Check sheet for the drawn part. Datum: minimum x, y, z corner. Units: mm. A direction names the side the tool comes from. Coordinates: 2 decimals unless noted, no trailing zeros. Write each loop counter-clockwise with the first axis right and the second up, starting at its lowest first coordinate (ties: lowest second). Pieces come first, ordered by that corner, then holes. Notation, with made-up numbers: M 84,11.5 L 107,11.5 A11 cw 107,15.5 Z; hole C 35,87 d10. An arc over 180 degrees is marked long. Answer in a Markdown table with one row per item.
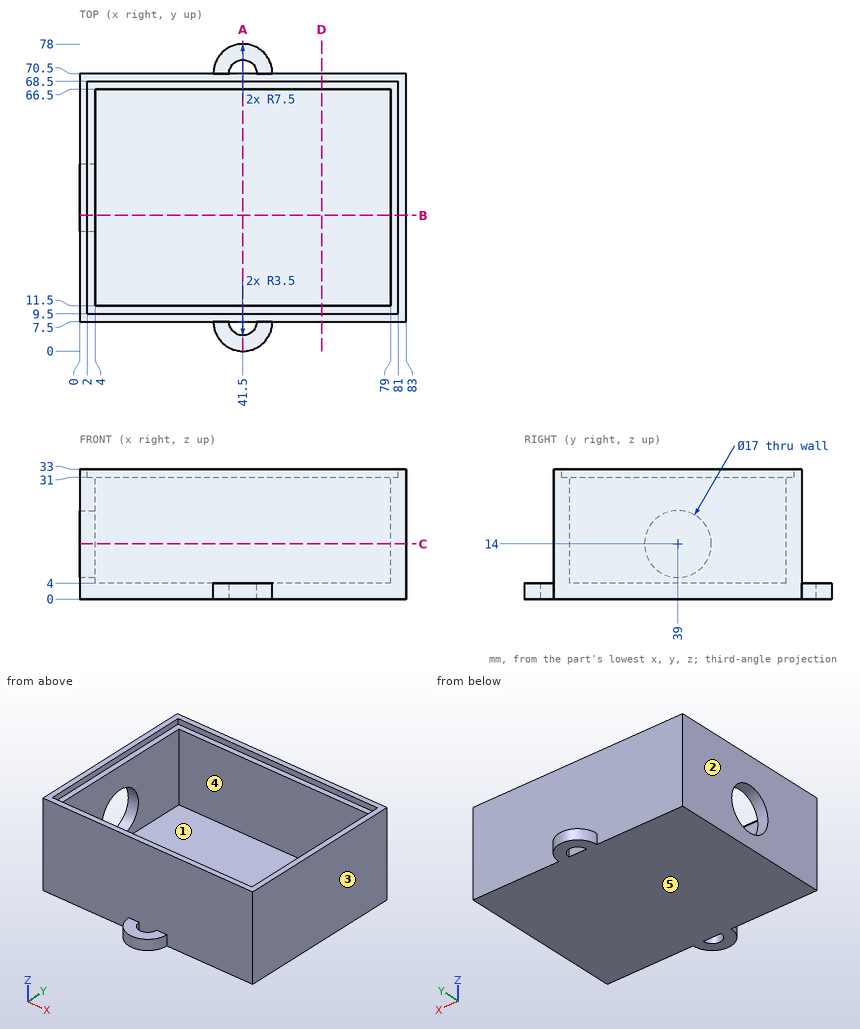
1) Sectioned sample at B-B (y = 34.5). Record the cut outline in (x, z).
Response values:
| item | result |
|---|---|
| outline | M 0,0 L 83,0 L 83,33 L 81,33 L 81,31 L 79,31 L 79,4 L 4,4 L 4,6.79 L 0,6.79 Z; M 0,21.21 L 4,21.21 L 4,31 L 2,31 L 2,33 L 0,33 Z |
2) Release check for a two-part mould opening along X. For the marked faces 3, 4 and 5 record: +X half, -X half, draft (parallel to the pull), parting line (faces both ways), or undercut.
Response values:
| item | result |
|---|---|
| face 3 | +X half |
| face 4 | undercut |
| face 5 | draft |
3) Tool access check on the marked faces 1 and 2. Record the directions out of +Z, -Z, +X, -X, +Y, -Y that give a thin tool (end or side, any length) a straight path to the whole face; none if there is none.
Response values:
| item | result |
|---|---|
| face 1 | +Z |
| face 2 | +Z, -Z, -X, +Y, -Y |
4) Sectioned sample at A-A (x = 41.5). Record the cut outline in (y, z), then the cut area to 3 significant figures.
Response values:
| item | result |
|---|---|
| outline | M 0,0 L 4,0 L 4,4 L 0,4 Z; M 7.5,0 L 70.5,0 L 70.5,33 L 68.5,33 L 68.5,31 L 66.5,31 L 66.5,4 L 11.5,4 L 11.5,31 L 9.5,31 L 9.5,33 L 7.5,33 Z; M 74,0 L 78,0 L 78,4 L 74,4 Z |
| area | 508 mm² |
5) Depth check by flat-ended pin: pin 1 (10 mm diameter, centred on x = 34.5, z = 21, fed in from +Y); pin 2 (8 mm diameter, centred on x = 26.5, y = 68, fed in from +Z); pin 3 (5 mm diameter, centred on x = 61, z = 10.5, fed in from -Y); pin 4 (4 mm diameter, centred on x = 9, y = 51, fed in from +Z). Enter the tip coordinate at first touch or a pass-through.
Response values:
| item | result |
|---|---|
| pin 1 | stops at y = 70.5 |
| pin 2 | stops at z = 33 |
| pin 3 | stops at y = 7.5 |
| pin 4 | stops at z = 4 |
6) Thickness scan on L1, parallel to Z at x = 1, y = 39; L2, parallel to X at y = 47, z = 7; L3, parallel to Y at x = 12, z = 28.5. Record the ranges inside material, lowest first. Write a range as [from, to].
Response values:
| item | result |
|---|---|
| L1 | z = [0, 5.5], [22.5, 33] |
| L2 | x = [0, 4], [79, 83] |
| L3 | y = [7.5, 11.5], [66.5, 70.5] |
7) Sectioned sample at C-C (z = 14). Record the cut outline in (x, y), then the cut area to 3 significant figures.
Response values:
| item | result |
|---|---|
| outline | M 0,7.5 L 83,7.5 L 83,70.5 L 0,70.5 L 0,47.5 L 4,47.5 L 4,66.5 L 79,66.5 L 79,11.5 L 4,11.5 L 4,30.5 L 0,30.5 Z |
| area | 1,040 mm² |
8) Sectioned sample at D-D (x = 61.5). Record the cut outline in (y, z).
Response values:
| item | result |
|---|---|
| outline | M 7.5,0 L 70.5,0 L 70.5,33 L 68.5,33 L 68.5,31 L 66.5,31 L 66.5,4 L 11.5,4 L 11.5,31 L 9.5,31 L 9.5,33 L 7.5,33 Z |
